Source: CAD feature listing. Evaluate the final solid. Frame: model axes, mm. Face numbers are marked on the shaded views. A direction names the side the tool comes from. Give positions to 0.01 mm unless a question says otherwise; leave off trailing zeros. Order: outer loops, then holes, each group sorted by start corner. A loop starts at its lowest first (then second) coordinate and runs counter-clockwise, first axis right, second up. Notation, with made-up numbers: M 87,83 L 113,83 A28 ccw 113,107 Z; hole C 78,-3.5 d10. An arc over 180 degrees is marked long. Use CSV: the item, a comma, the result in double quotes. Start each with the question number.
1. Reachability of the marked faces 1, 2, 3, 4 and 5 from +Z, -Z, +X, -X, +Y, -Y: full face, straight path, thin tool, end or side. Return the list, or none.
2. Pin query (flat end, axial travel): P1, Ø2, axis at x = 19.5, y = 25, coming from the +Z side; P2, Ø3, axis at x = 23, z = 9.5, coming from the +Y side; P3, Ø5, axis at x = 22, y = 22, coming from the +Z side. Return the tip coordinate at first contact, or that it passes through.
3. Section query A-A, the plane y = 22. State how many separate pieces and enclosed holes the cut face has, plus the area to 3 significant figures.
4. Line query: line 1 along Y through (x, z) = (22, 1.3); line 2 along Y through (x, z) = (8.5, 5); line 3 along Y through (x, z) = (33.5, 5). Output: solid intervals per line, ascending. Write a range as [from, to].
5. Mould query, pull axis Y, two halves, no side actions, for the marked faces 6, 7, 8 and 9. Classes: released by +Y, released by -Y, zero draft, split by the parting line, or undercut.
6. Section query C-C, the plane x = 31.8. Return the cut outline in (y, z).
7. Section query B-B, the plane z = 7. Return the cut outline in (x, y), plus the area to 3 significant figures.
from build123d import *

# Parameters (mm, degrees)
SKETCH_W        = 35.4
SKETCH_H        = 24
PAD_DEPTH       = 4
SKETCH001_W     = 35.4
SKETCH001_H     = 4
PAD001_DEPTH    = 16
SKETCH003_W     = 6
SKETCH003_H     = 10
PAD003_DEPTH    = 16
SKETCH004_R     = 1.4
POCKET_DEPTH    = 10
SKETCH005_W     = 6
SKETCH005_H     = 10
PAD004_DEPTH    = 16
SKETCH006_R     = 1.4
POCKET001_DEPTH = 10
SKETCH007_W     = 13
SKETCH007_H     = 4
PAD005_DEPTH    = 16
POCKET002_DEPTH = 2.4
SKETCH009_R     = 1.5
POCKET003_DEPTH = 5
POCKET004_DEPTH = 2
SKETCH011_R     = 1
POCKET005_DEPTH = 5
POCKET006_DEPTH = 2
SKETCH013_R     = 1
POCKET007_DEPTH = 5
FILLET_R        = 1
FILLET001_R     = 1
FILLET002_R     = 1
FILLET003_R     = 1
FILLET004_R     = 3
FILLET005_R     = 3
FILLET006_R     = 3
FILLET007_R     = 3


with BuildPart() as part:
    # Sketch → Pad (new body)
    with BuildSketch(Plane.XY):
        with Locations((17.7, 16)):
            Rectangle(SKETCH_W, SKETCH_H)
    extrude(amount=PAD_DEPTH)

    # Sketch001 → Pad001 (join)
    with BuildSketch(Plane.XY):
        with Locations((17.7, 2)):
            Rectangle(SKETCH001_W, SKETCH001_H)
    extrude(amount=PAD001_DEPTH)

    # Sketch003 → Pad003 (join)
    with BuildSketch(Plane.XY):
        with Locations((3, 18)):
            Rectangle(SKETCH003_W, SKETCH003_H)
    extrude(amount=PAD003_DEPTH)

    # Sketch004 (on Face14 of Pad003) → Pocket (cut)
    with BuildSketch(Plane(origin=(0, 23, 0), x_dir=(-1, 0, 0), z_dir=(0, 1, 0))):
        with Locations((-3.6, 10)):
            Circle(SKETCH004_R)
    extrude(amount=-POCKET_DEPTH, mode=Mode.SUBTRACT)

    # Sketch005 → Pad004 (join)
    with BuildSketch(Plane.XY):
        with Locations((32.4, 18)):
            Rectangle(SKETCH005_W, SKETCH005_H)
    extrude(amount=PAD004_DEPTH)

    # Sketch006 (on Face13 of Pad004) → Pocket001 (cut)
    with BuildSketch(Plane(origin=(0, 23, 0), x_dir=(-1, 0, 0), z_dir=(0, 1, 0))):
        with Locations((-31.8, 10)):
            Circle(SKETCH006_R)
    extrude(amount=-POCKET001_DEPTH, mode=Mode.SUBTRACT)

    # Sketch007 (on Face4 of Pocket001) → Pad005 (join)
    with BuildSketch(Plane(origin=(0, 0, 0), x_dir=(1, 0, 0), z_dir=(0, 0, -1))):
        with Locations((6.5, -30)):
            Rectangle(SKETCH007_W, SKETCH007_H)
    extrude(amount=-PAD005_DEPTH)

    # Sketch008 (on Face4 of Pad005) → Pocket002 (cut)
    with BuildSketch(Plane.XY.offset(4)):
        Polygon((12.72798, 20.425), (12.72798, 23.575), (10, 25.15), (7.27202, 23.575), (7.27202, 20.425), (10, 18.85), align=None)
        Polygon((24.72798, 20.425), (24.72798, 23.575), (22, 25.15), (19.27202, 23.575), (19.27202, 20.425), (22, 18.85), align=None)
        Polygon((12.72798, 11.575), (10, 13.15), (7.27202, 11.575), (7.27202, 8.425), (10, 6.85), (12.72798, 8.425), align=None)
        Polygon((24.72798, 8.425), (24.72798, 11.575), (22, 13.15), (19.27202, 11.575), (19.27202, 8.425), (22, 6.85), align=None)
    extrude(amount=-POCKET002_DEPTH, mode=Mode.SUBTRACT)

    # Sketch009 (on Face2 of Pocket002) → Pocket003 (cut)
    with BuildSketch(Plane(origin=(0, 0, 0), x_dir=(1, 0, 0), z_dir=(0, 0, -1))):
        with Locations((10, -10)):
            Circle(SKETCH009_R)
        with Locations((22, -10)):
            Circle(SKETCH009_R)
        with Locations((22, -22)):
            Circle(SKETCH009_R)
        with Locations((10, -22)):
            Circle(SKETCH009_R)
    extrude(amount=-POCKET003_DEPTH, mode=Mode.SUBTRACT)

    # Sketch010 (on Face25 of Pocket003) → Pocket004 (cut)
    with BuildSketch(Plane(origin=(0, 4, 0), x_dir=(-1, 0, 0), z_dir=(0, 1, 0))):
        Polygon((-3.051443, 8.875), (-3.051443, 11.125), (-5, 12.25), (-6.948557, 11.125), (-6.948557, 8.875), (-5, 7.75), align=None)
        Polygon((-21.751443, 8.875), (-21.751443, 11.125), (-23.7, 12.25), (-25.648557, 11.125), (-25.648557, 8.875), (-23.7, 7.75), align=None)
    extrude(amount=-POCKET004_DEPTH, mode=Mode.SUBTRACT)

    # Sketch011 (on Face55 of Pocket004) → Pocket005 (cut)
    with BuildSketch(Plane.XZ):
        with Locations((5, 10)):
            Circle(SKETCH011_R)
        with Locations((23.7, 10)):
            Circle(SKETCH011_R)
    extrude(amount=-POCKET005_DEPTH, mode=Mode.SUBTRACT)

    # Sketch012 (on Face18 of Pocket005) → Pocket006 (cut)
    with BuildSketch(Plane.XZ.offset(-28)):
        Polygon((6.948557, 11.125), (5, 12.25), (3.051443, 11.125), (3.051443, 8.875), (5, 7.75), (6.948557, 8.875), align=None)
    extrude(amount=-POCKET006_DEPTH, mode=Mode.SUBTRACT)

    # Sketch013 (on Face50 of Pocket006) → Pocket007 (cut)
    with BuildSketch(Plane(origin=(0, 32, 0), x_dir=(-1, 0, 0), z_dir=(0, 1, 0))):
        with Locations((-5, 10)):
            Circle(SKETCH013_R)
    extrude(amount=-POCKET007_DEPTH, mode=Mode.SUBTRACT)

    # Fillet
    fillet_edges = [part.edges().sort_by_distance(p)[0] for p in [
        (0, 18, 0),
    ]]
    fillet(fillet_edges, radius=FILLET_R)

    # Fillet001
    fillet001_edges = [part.edges().sort_by_distance(p)[0] for p in [
        (35.4, 18, 0),
    ]]
    fillet(fillet001_edges, radius=FILLET001_R)

    # Fillet002
    fillet002_edges = [part.edges().sort_by_distance(p)[0] for p in [
        (17.7, 0, 0),
    ]]
    fillet(fillet002_edges, radius=FILLET002_R)

    # Fillet003
    fillet003_edges = [part.edges().sort_by_distance(p)[0] for p in [
        (7, 32, 0),
    ]]
    fillet(fillet003_edges, radius=FILLET003_R)

    # Fillet004
    fillet004_edges = [part.edges().sort_by_distance(p)[0] for p in [
        (0, 18, 16),
    ]]
    fillet(fillet004_edges, radius=FILLET004_R)

    # Fillet005
    fillet005_edges = [part.edges().sort_by_distance(p)[0] for p in [
        (0, 29.5, 16),
    ]]
    fillet(fillet005_edges, radius=FILLET005_R)

    # Fillet006
    fillet006_edges = [part.edges().sort_by_distance(p)[0] for p in [
        (0, 2.5, 16),
    ]]
    fillet(fillet006_edges, radius=FILLET006_R)

    # Fillet007
    fillet007_edges = [part.edges().sort_by_distance(p)[0] for p in [
        (35.4, 18, 16),
    ]]
    fillet(fillet007_edges, radius=FILLET007_R)


solid = part.part
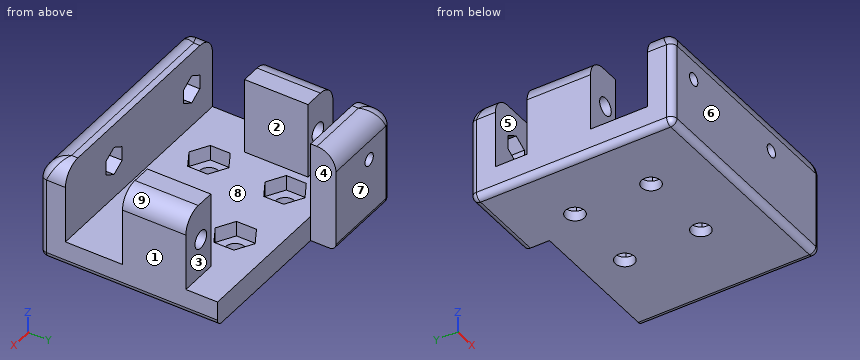
Result set:
1,face 1,"+Z, -Z, +X, +Y, -Y"
1,face 2,"+Z"
1,face 3,"+Z, +X, -X, +Y"
1,face 4,"+Z, -Z, +X, +Y"
1,face 5,"+Z, +X, -X"
2,P1,"z = 4"
2,P2,"y = 4"
2,P3,"z = 1.6"
3,separate pieces,"3"
3,enclosed holes,"2"
3,area,"233 mm2"
4,line 1,"[0, 8.5], [11.5, 20.5], [23.5, 28]"
4,line 2,"[0, 4], [28, 32]"
4,line 3,"[0, 4], [13, 23]"
5,face 6,"released by -Y"
5,face 7,"released by +Y"
5,face 8,"undercut"
5,face 9,"zero draft"
6,outline,"M 0,1 A1 ccw 1,0 L 28,0 L 28,4 L 23,4 L 23,8.6 L 13,8.6 L 13,4 L 4,4 L 4,16 L 3,16 A3 ccw 0,13 Z; M 13,11.4 L 23,11.4 L 23,16 L 13,16 Z"
7,outline,"M 0,1 A1 ccw 1,0 L 34.4,0 A1 ccw 35.4,1 L 35.4,4 L 0,4 Z; M 0,13 L 6,13 L 6,23 L 0,23 Z; M 0,28 L 13,28 L 13,32 L 1,32 A1 ccw 0,31 Z; M 29.4,13 L 35.4,13 L 35.4,23 L 29.4,23 Z"
7,area,"313 mm2"
